Design review of the part built by this model. Coordinates are the model's own, in mm. A direction names the side the tool comes from. Coordinates: 2 decimals unless noted, no trailing zeros. Write each loop counter-clockwise with the first axis right and the second up, starting at its lowest first coordinate (ties: lowest second). Pieces come first, ordered by that corner, then holes.
Q1. Add section A-A, the plane z = 0. Give the boundary of the cut face in (x, y), plus the area to 3 significant figures.
Q2. Add section D-D, the plane y = 11.5. Give the boundary of the cut face in (x, z), plus the area to 3 significant figures.
Q3. Clearance check with flat-ended pins moving along their axes: pin 1 Ø8 at (x, z) = (28, 7.5) entering from +Y; pin 2 Ø12 at (x, y) = (-20.5, 4) entering from +Z; pin 3 Ø12 at (x, y) = (17.5, 6.5) entering from -Z; pin 4 Ø10 at (x, z) = (14.5, -5) entering from -Y. State where each tip first meets the part, or that it passes through.
Q4. Add section B-B, the plane y = 3.75. Give the boundary of the cut face in (x, z).
Q5. To check wall thickness, follow probe 1 along Y at (x, z) = (1, 36); probe 2 along Z at (x, y) = (3, 0.5); probe 3 along Z at (x, y) = (-9.5, 3.5). State the ranges of each line that lie inside material, in increasing order.
Q6. Machinability: for faces 1 (the face through (30.318, 12.535, 17.488)), 2 (the face through (0, 13, -31)), 3 (the face through (29.427, -2.465, -14.973)), 4 (the face through (0, -2, 31)), 5 (the face through (-30.304, -2.465, 17.512)), which of the approach directions +Z, -Z, +X, -X, +Y, -Y give a long, thin tool a straight path to every point of the face, cutting with its end or side? Answer none if there is none.
Q7. The part is to be moulded in two halves that separate along Z. For faces 6 (the face through (-28, 15, -16)), 7 (the face through (-27.621, -2.465, 17.987)), 8 (the face through (1.39, 4.93, -24.97)), say which applies: +Z half, -Z half, draft (parallel to the pull), parting line (faces both ways), or undercut.
Q8. Add section C-C, the plane x = 6. Give the boundary of the cut face in (y, z).
from build123d import *

# Parameters (mm, degrees)
SKETCH1_R           = 40
BOSS_EXTRUDE1_DEPTH = 10
BOSS_EXTRUDE4_START = -10
BOSS_EXTRUDE4_DEPTH = 5
BOSS_EXTRUDE5_START = 5
BOSS_EXTRUDE5_DEPTH = 5


with BuildPart() as part:
    # Sketch1 → Boss-Extrude1 (new body)
    with BuildSketch(Plane(origin=(0, 0, 0), x_dir=(1, 0, 0), z_dir=(0, 1, 0))):
        with Locations(Location((0, 0, 0), (0, 0, 270))):
            Circle(SKETCH1_R)
        with BuildLine():
            Line((-2, 23.665639649), (-0.800587161, 26.237788783))
            ThreePointArc((-0.800587161, 26.237788783), (0, 26.25), (0.800587161, 26.237788783))
            Line((0.800587161, 26.237788783), (2, 23.665639649))
            ThreePointArc((2, 23.665639649), (11.875, 20.56810334), (19.495045133, 13.564870632))
            Line((19.495045133, 13.564870632), (22.322298044, 13.812223211))
            ThreePointArc((22.322298044, 13.812223211), (22.733166849, 13.125), (23.122885205, 12.425565572))
            Line((23.122885205, 12.425565572), (21.495045133, 10.100769017))
            ThreePointArc((21.495045133, 10.100769017), (23.75, 0), (21.495045133, -10.100769017))
            Line((21.495045133, -10.100769017), (23.122885205, -12.425565572))
            ThreePointArc((23.122885205, -12.425565572), (22.733166849, -13.125), (22.322298044, -13.812223211))
            Line((22.322298044, -13.812223211), (19.495045133, -13.564870632))
            ThreePointArc((19.495045133, -13.564870632), (11.875, -20.56810334), (2, -23.665639649))
            Line((2, -23.665639649), (0.800587161, -26.237788783))
            ThreePointArc((0.800587161, -26.237788783), (0, -26.25), (-0.800587161, -26.237788783))
            Line((-0.800587161, -26.237788783), (-2, -23.665639649))
            ThreePointArc((-2, -23.665639649), (-11.875, -20.56810334), (-19.495045133, -13.564870632))
            Line((-19.495045133, -13.564870632), (-22.322298044, -13.812223211))
            ThreePointArc((-22.322298044, -13.812223211), (-22.733166849, -13.125), (-23.122885205, -12.425565572))
            Line((-23.122885205, -12.425565572), (-21.495045133, -10.100769017))
            ThreePointArc((-21.495045133, -10.100769017), (-23.75, 0), (-21.495045133, 10.100769017))
            Line((-21.495045133, 10.100769017), (-23.122885205, 12.425565572))
            ThreePointArc((-23.122885205, 12.425565572), (-22.733166849, 13.125), (-22.322298044, 13.812223211))
            Line((-22.322298044, 13.812223211), (-19.495045133, 13.564870632))
            ThreePointArc((-19.495045133, 13.564870632), (-11.875, 20.56810334), (-2, 23.665639649))
        make_face(mode=Mode.SUBTRACT)
    extrude(amount=BOSS_EXTRUDE1_DEPTH)

    # 1,2,3 → Boss-Extrude4 (add)
    with BuildSketch(Plane(origin=(0, 10, 0), x_dir=(1, 0, 0), z_dir=(0, 1, 0)).offset(BOSS_EXTRUDE4_START)):
        with BuildLine():
            Line((2.5, 30.899029111), (1.012702288, 34.985345991))
            ThreePointArc((1.012702288, 34.985345991), (0, 35), (-1.012702288, 34.985345991))
            Line((-1.012702288, 34.985345991), (-2.5, 30.899029111))
            ThreePointArc((-2.5, 30.899029111), (0, 31), (2.5, 30.899029111))
        make_face()
        with BuildLine():
            Line((25.509344162, 17.614578065), (29.791847244, 18.369698903))
            ThreePointArc((29.791847244, 18.369698903), (30.310889132, 17.5), (30.804549532, 16.615647087))
            Line((30.804549532, 16.615647087), (28.009344162, 13.284451046))
            ThreePointArc((28.009344162, 13.284451046), (26.846787517, 15.5), (25.509344162, 17.614578065))
        make_face()
        with BuildLine():
            Line((28.009344162, -13.284451046), (30.804549532, -16.615647087))
            ThreePointArc((30.804549532, -16.615647087), (30.310889132, -17.5), (29.791847244, -18.369698903))
            Line((29.791847244, -18.369698903), (25.509344162, -17.614578065))
            ThreePointArc((25.509344162, -17.614578065), (26.846787517, -15.5), (28.009344162, -13.284451046))
        make_face()
        with BuildLine():
            Line((2.5, -30.899029111), (1.012702288, -34.985345991))
            ThreePointArc((1.012702288, -34.985345991), (0, -35), (-1.012702288, -34.985345991))
            Line((-1.012702288, -34.985345991), (-2.5, -30.899029111))
            ThreePointArc((-2.5, -30.899029111), (0, -31), (2.5, -30.899029111))
        make_face()
        with BuildLine():
            Line((-25.509344162, -17.614578065), (-29.791847244, -18.369698903))
            ThreePointArc((-29.791847244, -18.369698903), (-30.310889132, -17.5), (-30.804549532, -16.615647087))
            Line((-30.804549532, -16.615647087), (-28.009344162, -13.284451046))
            ThreePointArc((-28.009344162, -13.284451046), (-26.846787517, -15.5), (-25.509344162, -17.614578065))
        make_face()
        with BuildLine():
            Line((-28.009344162, 13.284451046), (-30.804549532, 16.615647087))
            ThreePointArc((-30.804549532, 16.615647087), (-30.310889132, 17.5), (-29.791847244, 18.369698903))
            Line((-29.791847244, 18.369698903), (-25.509344162, 17.614578065))
            ThreePointArc((-25.509344162, 17.614578065), (-26.846787517, 15.5), (-28.009344162, 13.284451046))
        make_face()
    extrude(amount=-BOSS_EXTRUDE4_DEPTH)

    # 1,2,3<2> → Boss-Extrude5 (add)
    with BuildSketch(Plane(origin=(0, 10, 0), x_dir=(1, 0, 0), z_dir=(0, 1, 0)).offset(BOSS_EXTRUDE5_START)):
        with BuildLine():
            Line((2.5, 30.899029111), (1.012702288, 34.985345991))
            ThreePointArc((1.012702288, 34.985345991), (0, 35), (-1.012702288, 34.985345991))
            Line((-1.012702288, 34.985345991), (-2.5, 30.899029111))
            ThreePointArc((-2.5, 30.899029111), (0, 31), (2.5, 30.899029111))
        make_face()
        with BuildLine():
            Line((25.509344162, 17.614578065), (29.791847244, 18.369698903))
            ThreePointArc((29.791847244, 18.369698903), (30.310889132, 17.5), (30.804549532, 16.615647087))
            Line((30.804549532, 16.615647087), (28.009344162, 13.284451046))
            ThreePointArc((28.009344162, 13.284451046), (26.846787517, 15.5), (25.509344162, 17.614578065))
        make_face()
        with BuildLine():
            Line((28.009344162, -13.284451046), (30.804549532, -16.615647087))
            ThreePointArc((30.804549532, -16.615647087), (30.310889132, -17.5), (29.791847244, -18.369698903))
            Line((29.791847244, -18.369698903), (25.509344162, -17.614578065))
            ThreePointArc((25.509344162, -17.614578065), (26.846787517, -15.5), (28.009344162, -13.284451046))
        make_face()
        with BuildLine():
            Line((2.5, -30.899029111), (1.012702288, -34.985345991))
            ThreePointArc((1.012702288, -34.985345991), (0, -35), (-1.012702288, -34.985345991))
            Line((-1.012702288, -34.985345991), (-2.5, -30.899029111))
            ThreePointArc((-2.5, -30.899029111), (0, -31), (2.5, -30.899029111))
        make_face()
        with BuildLine():
            Line((-25.509344162, -17.614578065), (-29.791847244, -18.369698903))
            ThreePointArc((-29.791847244, -18.369698903), (-30.310889132, -17.5), (-30.804549532, -16.615647087))
            Line((-30.804549532, -16.615647087), (-28.009344162, -13.284451046))
            ThreePointArc((-28.009344162, -13.284451046), (-26.846787517, -15.5), (-25.509344162, -17.614578065))
        make_face()
        with BuildLine():
            Line((-28.009344162, 13.284451046), (-30.804549532, 16.615647087))
            ThreePointArc((-30.804549532, 16.615647087), (-30.310889132, 17.5), (-29.791847244, 18.369698903))
            Line((-29.791847244, 18.369698903), (-25.509344162, 17.614578065))
            ThreePointArc((-25.509344162, 17.614578065), (-26.846787517, 15.5), (-28.009344162, 13.284451046))
        make_face()
    extrude(amount=-BOSS_EXTRUDE5_DEPTH)


solid = part.part
Here are the results:
1. outline: (-40, 0) - (-23.75, 0) - (-23.75, 10) - (-40, 10) - close; (23.75, 0) - (40, 0) - (40, 10) - (23.75, 10) - close
1. area: 325 mm2
2. outline: (-30.8, -16.62) arc R35 ccw to (-29.79, -18.37) - (-25.51, -17.61) arc R31 cw to (-28.01, -13.28) - close; (-30.8, 16.62) - (-28.01, 13.28) arc R31 cw to (-25.51, 17.61) - (-29.79, 18.37) arc R35 ccw to start; (-2.5, -30.9) - (-1.01, -34.99) arc R35 ccw to (1.01, -34.99) - (2.5, -30.9) arc R31 cw to start; (-2.5, 30.9) arc R31 cw to (2.5, 30.9) - (1.01, 34.99) arc R35 ccw to (-1.01, 34.99) - close; (25.51, -17.61) - (29.79, -18.37) arc R35 ccw to (30.8, -16.62) - (28.01, -13.28) arc R31 cw to start; (25.51, 17.61) arc R31 cw to (28.01, 13.28) - (30.8, 16.62) arc R35 ccw to (29.79, 18.37) - close
2. area: 84.2 mm2
3. pin 1: stops at y = 10
3. pin 2: stops at z = 37.28
3. pin 3: stops at z = -38.31
3. pin 4: passes through
4. outline: circle Ø80 at (0, 0); hole (-23.12, -12.43) arc R26.25 ccw to (-22.32, -13.81) - (-19.5, -13.56) arc R23.75 ccw to (-2, -23.67) - (-0.8, -26.24) arc R26.25 ccw to (0.8, -26.24) - (2, -23.67) arc R23.75 ccw to (19.5, -13.56) - (22.32, -13.81) arc R26.25 ccw to (23.12, -12.43) - (21.5, -10.1) arc R23.75 ccw to (21.5, 10.1) - (23.12, 12.43) arc R26.25 ccw to (22.32, 13.81) - (19.5, 13.56) arc R23.75 ccw to (2, 23.67) - (0.8, 26.24) arc R26.25 ccw to (-0.8, 26.24) - (-2, 23.67) arc R23.75 ccw to (-19.5, 13.56) - (-22.32, 13.81) arc R26.25 ccw to (-23.12, 12.43) - (-21.5, 10.1) arc R23.75 ccw to (-21.5, -10.1) - close
5. probe 1: y = 0 to 10
5. probe 2: z = -39.89 to -23.56, 23.56 to 39.89
5. probe 3: z = -38.86 to -21.77, 21.77 to 38.86
6. face 1: +Z, +X, +Y
6. face 2: +Y
6. face 3: +X, -Y
6. face 4: -Y
6. face 5: +Z, -X, -Y
7. face 6: draft
7. face 7: +Z half
7. face 8: undercut
8. outline: (0, -39.55) - (10, -39.55) - (10, -22.98) - (0, -22.98) - close; (0, 22.98) - (10, 22.98) - (10, 39.55) - (0, 39.55) - close
